For this review, use the dimensioned drawing (mm, ordinates from the lowest corner) and the shaded views. Round coordinates to 2 decimals unless told otherwise and drop trailing zeros. Order: outer loops, then holes, each group sorted by start corner. A loop starts at its lowest first (then second) coordinate and runs counter-clockwise, first axis right, second up. Notation, with made-up numbers: (-36, 21) - (-32, 21) arc R34 ccw to (-32, 52) - close; hole circle Ø6 at (-6.75, 75). An arc over 180 degrees is marked (long way). Write item = value, one per line.
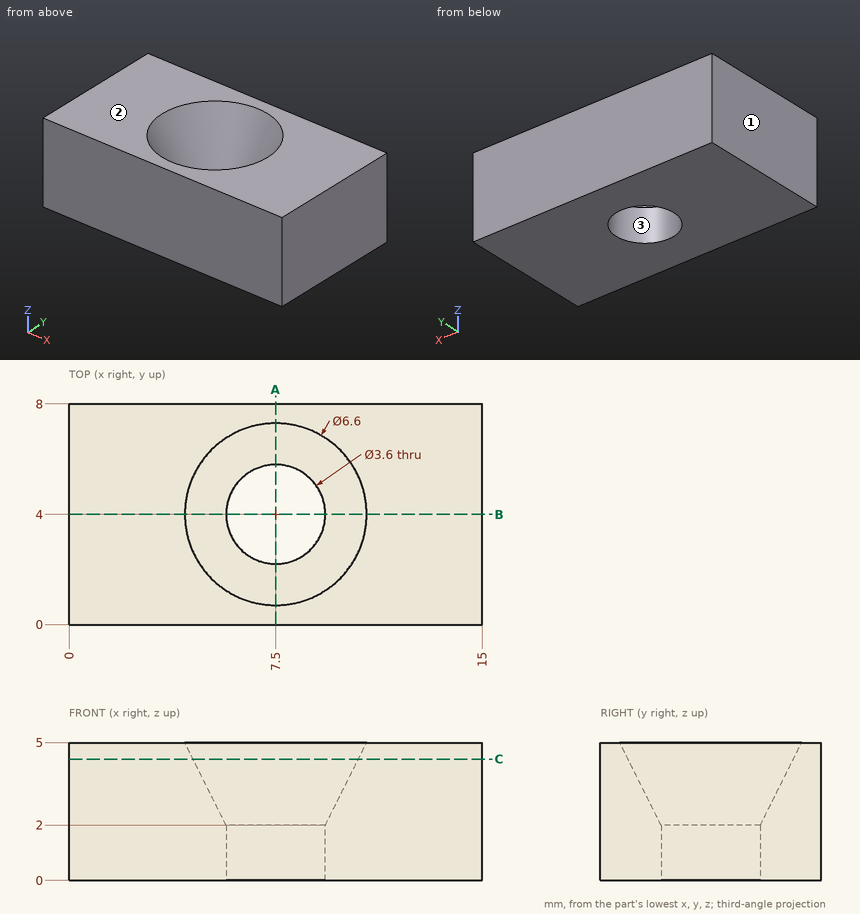
Item 1: For line 1 along Y through (x, z) = (7.5, 1.4); line 2 along X through (y, z) = (2.75, 4.35); line 3 along X through (y, z) = (4.25, 3), list the stretches that pass through material, from the lowest coordinate up. Write a range as [from, to].
Data:
line_1 = [0, 2.2], [5.8, 8]
line_2 = [0, 4.8], [10.2, 15]
line_3 = [0, 5.21], [9.79, 15]
Item 2: Insertion check: P1, Ø3, axis at x = 7.5, y = 4, coming from the -Z side. The pin has a flat end and moves straight along its axis. Give the tip position at first contact, or say it passes through.
Data:
P1 = through
Item 3: Take a section at C-C, the plane z = 4.4. State the section outline as (x, y) points.
Data:
outline = (0, 0) - (15, 0) - (15, 8) - (0, 8) - close; hole circle Ø6 at (7.5, 4)
Item 4: Take a section at A-A, the plane x = 7.5. State the section outline as (y, z) points, and give its area (3 significant figures).
Data:
outline = (0, 0) - (2.2, 0) - (2.2, 2) - (0.7, 5) - (0, 5) - close; (5.8, 0) - (8, 0) - (8, 5) - (7.3, 5) - (5.8, 2) - close
area = 17.5 mm2
Item 5: Take a section at B-B, the plane y = 4. State the section outline as (x, z) points.
Data:
outline = (0, 0) - (5.7, 0) - (5.7, 2) - (4.2, 5) - (0, 5) - close; (9.3, 0) - (15, 0) - (15, 5) - (10.8, 5) - (9.3, 2) - close
Item 6: The part is to be moulded in two halves that separate along X. For the marked faces 1, 2 and 3, say which applies: +X half, -X half, draft (parallel to the pull), parting line (faces both ways), or undercut.
Data:
face_1 = -X half
face_2 = draft
face_3 = undercut
